Part model, mm, in its own coordinate system. A direction names the side the tool comes from. Give positions to 0.01 mm unless a question says otherwise; leave off trailing zeros. Order: outer loops, then holes, each group sorted by start corner. A loop starts at its lowest first (then second) coordinate and runs counter-clockwise, first axis right, second up. Notation, with made-up numbers: M 52.25,53 L 89.25,53 A19 ccw 89.25,74 Z; hole C 45,29 d1. An arc over 180 degrees is marked long. Return JSON: item names as keys, results as strings.
from build123d import *

# Parameters (mm, degrees)
F0_W           = 28.5
F0_H           = 27.5
F1_DEPTH       = 1.5
F2_R           = 8
F3_R           = 1.5
F4_DEPTH       = 15.5
F5_W           = 11.5
F5_H           = 11.5
F6_DEPTH       = 3
F8_DEPTH       = 11.5
F9_R           = 1.2194434125
F10_R          = 0.25
F11_W          = 13
F11_H          = 13
F11_R          = 5.5650544151
F12_DEPTH      = 3
F13_DEPTH      = 8
F14_W          = 5
F14_H          = 13
F15_DEPTH      = 8
F15_DEPTH_BACK = 3
F16_W          = 11
F16_H          = 10
F17_DEPTH      = 1


with BuildPart() as f1:
    # F0 (on Top) → F1 (new body)
    with BuildSketch(Plane.XY):
        Rectangle(F0_W, F0_H)
    extrude(amount=F1_DEPTH)

    # F2
    f2_edges = [f1.edges().sort_by_distance(p)[0] for p in [
        (14.25, -13.75, 0.75),
        (-14.25, -13.75, 0.75),
    ]]
    fillet(f2_edges, radius=F2_R)

    # F3 (on face) → F4 (join)
    with BuildSketch(Plane.XY.offset(1.5)):
        with Locations((5.25, 7.75)):
            Circle(F3_R)
    extrude(amount=F4_DEPTH)

    # F5 (on face) → F6 (join)
    with BuildSketch(Plane.XY.offset(1.5)):
        with Locations((7.5, -3)):
            Rectangle(F5_W, F5_H)
    extrude(amount=F6_DEPTH)

    # F7 (on face) → F8 (join)
    with BuildSketch(Plane.XY.offset(4.5)):
        with BuildLine():
            ThreePointArc((10.75, -3), (9.7980970389, -0.7019029611), (7.5, 0.25))
            Line((7.5, 0.25), (7.5, -6.25))
            ThreePointArc((7.5, -6.25), (9.7980970389, -5.2980970389), (10.75, -3))
        make_face()
        with BuildLine():
            Line((7.5, -6.25), (7.5, 0.25))
            ThreePointArc((7.5, 0.25), (4.25, -3), (7.5, -6.25))
        make_face()
    extrude(amount=F8_DEPTH)

    # F9
    f9_edges = [f1.edges().sort_by_distance(p)[0] for p in [
        (3.75, 7.75, 17),
    ]]
    fillet(f9_edges, radius=F9_R)

    # F10
    f10_edges = [f1.edges().sort_by_distance(p)[0] for p in [
        (4.25, -3, 16),
    ]]
    fillet(f10_edges, radius=F10_R)

    # F11 (on face) → F12 (join)
    with BuildSketch(Plane.XY.offset(1.5)):
        with Locations((-6.75, -1.75)):
            Rectangle(F11_W, F11_H)
        with Locations((-6.75, -1.75)):
            Circle(F11_R, mode=Mode.SUBTRACT)
    extrude(amount=F12_DEPTH)

    # F13 (add): a face of the model
    f13_faces = [f1.faces().sort_by_distance(p)[0] for p in [
        (-6.75, -1.75, 1.5),
    ]]
    extrude(f13_faces, amount=F13_DEPTH)

    # F14 (on face) → F15 (join, two sides)
    with BuildSketch(Plane.XY.offset(9.5)) as f15_sk:
        with Locations((-7.75, -1.75)):
            Rectangle(F14_W, F14_H)
    extrude(amount=-F15_DEPTH)
    extrude(f15_sk.sketch, amount=F15_DEPTH_BACK)

    # F16 (on face) → F17 (join)
    with BuildSketch(Plane.XY.offset(9.5)):
        with Locations((-6.75, -1.75)):
            Rectangle(F16_W, F16_H)
    extrude(amount=F17_DEPTH)


solid = f1.part
Q1. Band-saw the part on D-D (x = 2.75). Give the cut face in (y, z).
Established:
{"outline": "M -13.75,0 L 13.75,0 L 13.75,1.5 L 2.75,1.5 L 2.75,4.5 L -8.75,4.5 L -8.75,1.5 L -13.75,1.5 Z"}
Q2. Pin check, flat tips, straight feed: pin 1 (0.9 mm diameter, centred on y = -5, z = 2.5, fed in from +X); pin 2 (4 mm diameter, centred on x = 9, y = -5, fed in from +Z); pin 3 (4 mm diameter, centred on y = -2.5, z = 10.5, fed in from +X). Stop position of each tip, or through.
Established:
{"pin 1": "stops at x = 13.25", "pin 2": "stops at z = 16", "pin 3": "stops at x = 10.75"}
Q3. Two-plate mould, pull along Z, no slides. Class faces 1 (the flat face through (7, -3, 16)), 2 (the flat face through (7, 2.75, 3)), 3 (the flat face through (-11, -6, 9.5)): +Z half, -Z half, draft (parallel to the pull), parting line (faces both ways), or undercut.
Established:
{"face 1": "+Z half", "face 2": "draft", "face 3": "undercut"}
Q4. Band-saw the part on C-C (y = 10.75). Give the cut face in (x, z), then the cut area to 4 significant figures.
Established:
{"outline": "M -14.25,0 L 14.25,0 L 14.25,1.5 L -14.25,1.5 Z", "area": "42.75 mm²"}
Q5. 3-axis set-ups, long thin cutter, end or side, ignore diameter. For faces 4 (the flat face through (-3, -6.75, 10)), 5 (the flat face through (-1.25, -2, 10)), 6 (the flat face through (-11, -6.75, 10)), 7 (the cylindrical face through (-1.186, -1.851, 6.965)): which of +Z, -Z, +X, -X, +Y, -Y reach the whole face in a straight line?
Established:
{"face 4": "+Z, +X, -Y", "face 5": "+Z, +Y, -Y", "face 6": "+Z, -X, -Y", "face 7": "none"}
Q6. Probe line 1 along X through (y, z) = (-7.25, 2); line 2 along Y through (x, z) = (12.5, 2.5); line 3 along Z through (x, y) = (-7.25, 10.5). List the from-to ranges inside material, lowest first.
Established:
{"line 1": "x = -13.25 to -0.25, 1.75 to 13.25", "line 2": "y = -8.75 to 2.75", "line 3": "z = 0 to 1.5"}
Q7. Band-saw the part on A-A (z = 6.25). Give the cut face in (x, y), then the cut area to 3 significant figures.
Established:
{"outline": "M -10.25,-8.25 L -5.25,-8.25 L -5.25,-7.11 A5.57 ccw -5.25,3.61 L -5.25,4.75 L -10.25,4.75 L -10.25,2.58 A5.57 ccw -10.25,-6.08 Z; C 5.25,7.75 d3; C 7.5,-3 d6.5", "area": "150 mm²"}
Q8. Band-saw the part on B-B (x = -3.25). Give the cut face in (y, z).
Established:
{"outline": "M -13.75,0 L 13.75,0 L 13.75,1.5 L 4.75,1.5 L 4.75,4.5 L 2.58,4.5 L 2.58,9.5 L 3.25,9.5 L 3.25,10.5 L -6.75,10.5 L -6.75,9.5 L -6.08,9.5 L -6.08,4.5 L -8.25,4.5 L -8.25,1.5 L -13.75,1.5 Z"}
